The listing builds one solid part. Answer for the finished solid, in the listing's coordinates (mm). Coordinates: 2 decimals unless noted, no trailing zeros. Order: outer loops, then holes, each group sorted by start corner. A loop starts at its lowest first (then second) coordinate and runs counter-clockwise, first axis right, second up. Notation, with made-up numbers: (30, -19) -> (75, -19) arc R26 ccw to (75, -1) -> close; hole circle Ø5 at (-19, 44). An arc over 180 degrees is marked (long way). Return JSON: item names as keys, results as strings.
```python
from build123d import *

# Parameters (mm, degrees)
BOSS_EXTRUDE1_DEPTH = 5
CUT_EXTRUDE1_REACH  = 7
SKETCH2_R           = 1


with BuildPart() as part:
    # Sketch1 → Boss-Extrude1 (new body)
    with BuildSketch(Plane(origin=(0, 0, 0), x_dir=(1, 0, 0), z_dir=(0, 1, 0))):
        with BuildLine():
            Line((0, -2.5), (-65, -2.5))
            ThreePointArc((-65, -2.5), (-67.5, 0), (-65, 2.5))
            Line((-65, 2.5), (0, 2.5))
            ThreePointArc((0, 2.5), (2.5, 0), (0, -2.5))
        make_face()
    extrude(amount=BOSS_EXTRUDE1_DEPTH)

    # Sketch2 → Cut-Extrude1 (cut, up to next)
    with BuildSketch(Plane(origin=(0, 5, 0), x_dir=(1, 0, 0), z_dir=(0, 1, 0)), mode=Mode.PRIVATE) as cut_extrude1_sk1:
        with Locations((-65, 0)):
            Circle(SKETCH2_R)
    cut_extrude1_tool1 = extrude(cut_extrude1_sk1.sketch, amount=-CUT_EXTRUDE1_REACH, mode=Mode.PRIVATE) & part.part
    add(cut_extrude1_tool1.solids().sort_by_distance((-65, 5, 0))[0], mode=Mode.SUBTRACT)
    # Sketch2 → Cut-Extrude1 (cut, up to next)
    with BuildSketch(Plane(origin=(0, 5, 0), x_dir=(1, 0, 0), z_dir=(0, 1, 0)), mode=Mode.PRIVATE) as cut_extrude1_sk2:
        Circle(SKETCH2_R)
    cut_extrude1_tool2 = extrude(cut_extrude1_sk2.sketch, amount=-CUT_EXTRUDE1_REACH, mode=Mode.PRIVATE) & part.part
    add(cut_extrude1_tool2.solids().sort_by_distance((0, 5, 0))[0], mode=Mode.SUBTRACT)


solid = part.part
```
Item 1: Flat-ended cylindrical pins translate along their axes: pin 1 (2.5 mm diameter, centred on x = -65, z = 0, fed in from +Y); pin 2 (2 mm diameter, centred on y = 2.5, z = 1.5, fed in from -X). Find the tip coordinate at first contact, or state that the pin passes through.
Answer list:
{"pin 1": "y = 5", "pin 2": "x = -67.45"}
Item 2: The part is cut by section B-B on y = 2.5. Determine the outline of the cut face in (x, z), plus the area to 3 significant figures.
Answer list:
{"outline": "(-65, -2.5) -> (0, -2.5) arc R2.5 ccw to (0, 2.5) -> (-65, 2.5) arc R2.5 ccw to start; hole circle Ø2 at (-65, 0); hole circle Ø2 at (0, 0)", "area": "338 mm2"}
Item 3: The part is cut by section A-A on z = 0. Determine the outline of the cut face in (x, y).
Answer list:
{"outline": "(-67.5, 0) -> (-66, 0) -> (-66, 5) -> (-67.5, 5) -> close; (-64, 0) -> (-1, 0) -> (-1, 5) -> (-64, 5) -> close; (1, 0) -> (2.5, 0) -> (2.5, 5) -> (1, 5) -> close"}
Item 4: Find the intervals of material crossed by probe 1 along X at (y, z) = (1.1, 0.05); probe 2 along X at (y, z) = (3.45, -0.4); probe 3 along Z at (x, y) = (-65, 1), in increasing order.
Answer list:
{"probe 1": "-67.5 to -66, -64 to -1, 1 to 2.5", "probe 2": "-67.47 to -65.92, -64.08 to -0.92, 0.92 to 2.47", "probe 3": "-2.5 to -1, 1 to 2.5"}
